Here's the drawing with two shaded views (mm, measured from the low corner). I have some questions. A direction names the side the tool comes from. Give positions to 0.01 mm unless a question says otherwise; leave off trailing zeros. Loops run counter-clockwise (first coordinate to the right, second up) from the corner with the lowest first, then second, coordinate; pieces in that order, holes last. Notation, with made-up numbers: (63, -19) - (88, -19) arc R20 ccw to (88, -11) - close; hole circle Ø3 at (-3, -10.75). An arc over 180 degrees is marked (long way). Use one line per item in the form item = value.
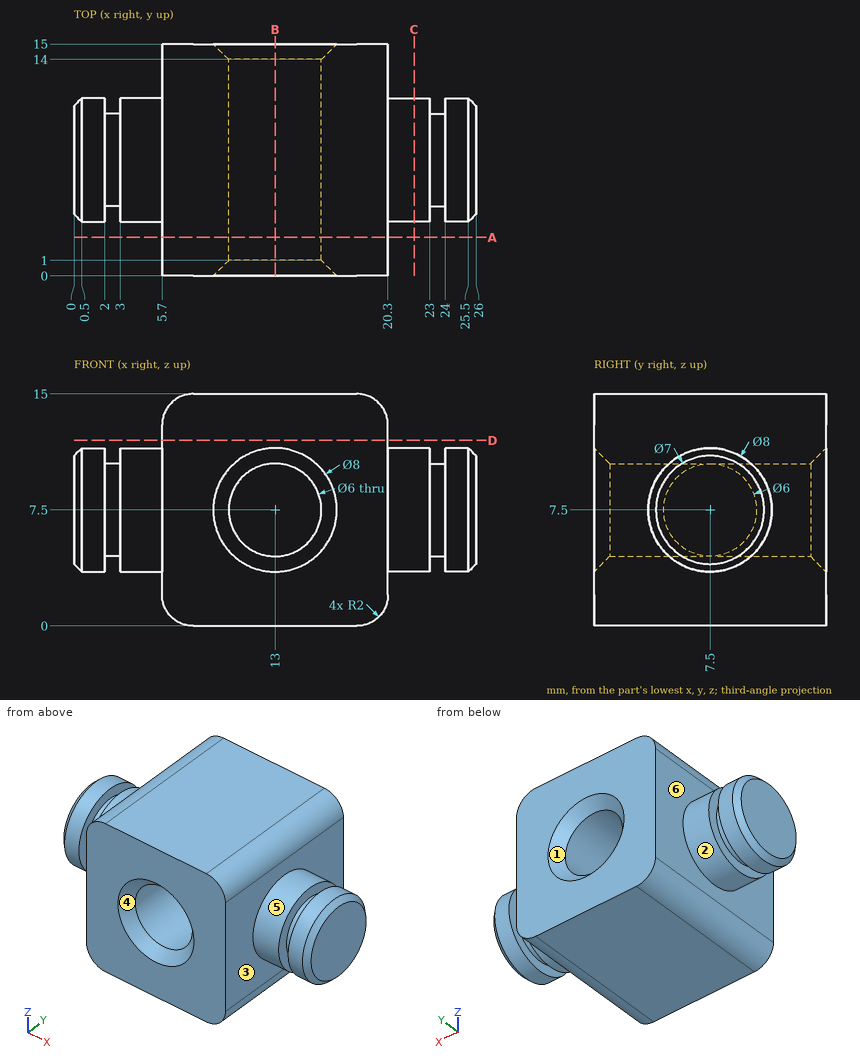
(1) Thinking about a two-plate mould opening in X: for the marked faces 4, 5 and 6, which applies, pulls with the +X half, pulls with the -X half, needs draft (parallel to the pull), parting line crosses it, or undercut?
Geometry says:
face_4 = undercut
face_5 = needs draft
face_6 = pulls with the -X half
(2) If I drill on probe 1 along Z at (x, y) = (13, 10.5); probe 2 along X at (y, z) = (6, 2.5); probe 3 along Z at (x, y) = (15.5, 13.25), over which ranges is the centre line in solid material (lowest first)?
Geometry says:
probe_1 = 0 to 4.5, 10.5 to 15
probe_2 = 5.7 to 20.3
probe_3 = 0 to 5.84, 9.16 to 15
(3) If we section it at C-C (x = 22): List the corners of the cut face in (y, z) for me, plus the area to 3 significant figures.
Geometry says:
outline = circle Ø8 at (7.5, 7.5)
area = 50.3 mm²
(4) If we section it at D-D (z = 12): List the corners of the cut face in (x, y) for me.
Geometry says:
outline = (5.7, 0) - (20.3, 0) - (20.3, 15) - (5.7, 15) - close
(5) If we section it at A-A (y = 2.5): List the corners of the cut face in (x, z) for me.
Geometry says:
outline = (5.7, 2) arc R2 ccw to (7.7, 0) - (18.3, 0) arc R2 ccw to (20.3, 2) - (20.3, 13) arc R2 ccw to (18.3, 15) - (7.7, 15) arc R2 ccw to (5.7, 13) - close; hole circle Ø6 at (13, 7.5)
(6) If we section it at B-B (x = 13): List the corners of the cut face in (y, z) for me, plus the area to 3 significant figures.
Geometry says:
outline = (0, 0) - (15, 0) - (15, 3.5) - (14, 4.5) - (1, 4.5) - (0, 3.5) - close; (0, 11.5) - (1, 10.5) - (14, 10.5) - (15, 11.5) - (15, 15) - (0, 15) - close
area = 133 mm²
(7) For the marked faces 1, 2 and 3, which set-ups out of +Z, -Z, +X, -X, +Y, -Y let a thin tool reach every point of the face, with its end or its side?
Geometry says:
face_1 = +Y
face_2 = -X
face_3 = +X
(8) For P1, Ø2, axis at x = 4.5, y = 6.5, coming from the +Z side, with a flat end and sliding along its axis, tell me the tip position at first contact or that it passes through.
Geometry says:
P1 = 11.5
